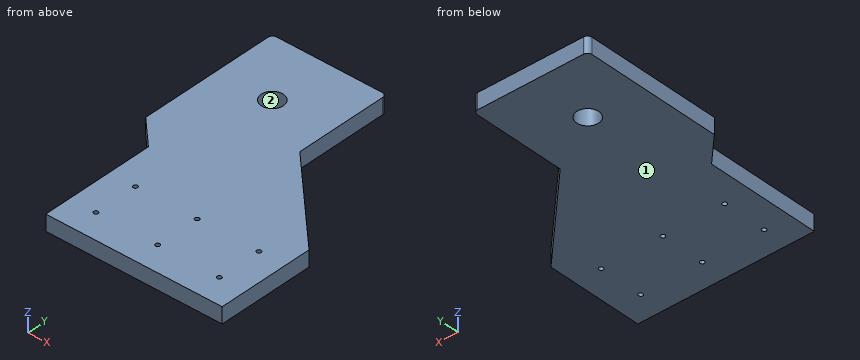
```python
from build123d import *

# Parameters (mm, degrees)
SKETCH1_R                      = 12.5
BOSS_EXTRUDE1_DEPTH            = 18
HOLE_FOR_M5_300_SC_NUTS_SP_1_D = 5


with BuildPart() as part:
    # Sketch1 → Boss-Extrude1 (new body)
    with BuildSketch(Plane.XY):
        with BuildLine():
            Line((4.070181983, 148.487708827), (4.070181983, 43.487708827))
            Line((4.070181983, 43.487708827), (104.070181983, -56.512291173))
            Line((104.070181983, -56.512291173), (104.070181983, -166.512291173))
            Line((104.070181983, -166.512291173), (-95.929818017, -166.512291173))
            Line((-95.929818017, -166.512291173), (-95.929818017, -36.512291173))
            Line((-95.929818017, -36.512291173), (-125.929818017, -6.512291173))
            Line((-125.929818017, -6.512291173), (-125.929818017, 148.487708827))
            ThreePointArc((-125.929818017, 148.487708827), (-124.465351923, 152.023242733), (-120.929818017, 153.487708827))
            Line((-120.929818017, 153.487708827), (-95.929818017, 153.487708827))
            Line((-95.929818017, 153.487708827), (-0.929818017, 153.487708827))
            ThreePointArc((-0.929818017, 153.487708827), (2.605715889, 152.023242733), (4.070181983, 148.487708827))
        make_face()
        with Locations((-62.929818017, 83.487708827)):
            Circle(SKETCH1_R, mode=Mode.SUBTRACT)
    extrude(amount=BOSS_EXTRUDE1_DEPTH)

    # Hole for M5 300® SC Nuts (SP)1 (through all)
    with Locations(Plane.XY.offset(18)):
        with Locations((74.070181983, -86.512291173), (74.070181983, -136.512291173), (4.070181983, -136.512291173), (-65.929818017, -136.512291173), (-65.929818017, -86.512291173), (4.070181983, -86.512291173)):
            Hole(HOLE_FOR_M5_300_SC_NUTS_SP_1_D / 2)


solid = part.part
```
Input: part model. Units: mm. Frame: model coordinates. Face numbers are marked on the shaded views. Give positions to 0.01 mm unless a question says otherwise; leave off trailing zeros. Order: outer loops, then holes, each group sorted by start corner. A loop starts at its lowest first (then second) coordinate and runs counter-clockwise, first axis right, second up. Notation, with made-up numbers: M -37.75,24.5 L -17.75,24.5 A4 cw -17.75,31.5 Z; hole C 13.25,78.25 d6. An arc over 180 degrees is marked long. Return JSON: item names as keys, results as strings.
1) Section query D-D on x = -100.5. Output: boundary loops of the cut face in (y, z), and give its area (3 significant figures).
Taken from the geometry:
{"outline": "M -31.94,0 L 153.49,0 L 153.49,18 L -31.94,18 Z", "area": "3,340 mm2"}
2) Section query C-C on y = -113. Output: boundary loops of the cut face in (x, z).
Taken from the geometry:
{"outline": "M -95.93,0 L 104.07,0 L 104.07,18 L -95.93,18 Z"}
3) Line query: L1, parallel to X at y = -135, z = 11.5; L2, parallel to Y at x = -64, z = 5; L3, parallel to X at y = -71.5, z = 10. Output: solid intervals per line, ascending. Write a range as [from, to].
Taken from the geometry:
{"L1": "x = [-95.93, -67.92], [-63.94, 2.08], [6.06, 72.08], [76.06, 104.07]", "L2": "y = [-166.51, -138.1], [-134.92, -88.1], [-84.92, 71.03], [95.94, 153.49]", "L3": "x = [-95.93, 104.07]"}
4) Section query B-B on z = 10.5. Output: boundary loops of the cut face in (x, y).
Taken from the geometry:
{"outline": "M -125.93,-6.51 L -95.93,-36.51 L -95.93,-166.51 L 104.07,-166.51 L 104.07,-56.51 L 4.07,43.49 L 4.07,148.49 A5 ccw -0.93,153.49 L -120.93,153.49 A5 ccw -125.93,148.49 Z; hole C -62.93,83.49 d25; hole C -65.93,-136.51 d5; hole C -65.93,-86.51 d5; hole C 4.07,-136.51 d5; hole C 4.07,-86.51 d5; hole C 74.07,-136.51 d5; hole C 74.07,-86.51 d5"}
5) Mould query, pull axis X, two halves, no side actions, for the marked faces 1 and 2. Classes: released by +X, released by -X, zero draft, split by the parting line, or undercut.
Taken from the geometry:
{"face 1": "zero draft", "face 2": "undercut"}
6) Contact query for flat-ended pins moving along their axis: pin 1 (15 mm diameter, centred on x = -62.93, y = 83.49, fed in from -Z); pin 2 (1.5 mm diameter, centred on y = 19.5, z = 10, fed in from +X); pin 3 (10 mm diameter, centred on y = -130, z = 9, fed in from -X). Output: stop coordinate, or through.
Taken from the geometry:
{"pin 1": "passes through", "pin 2": "stops at x = 28.81", "pin 3": "stops at x = -95.93"}
7) Section query A-A on y = 87. Output: boundary loops of the cut face in (x, z).
Taken from the geometry:
{"outline": "M -125.93,0 L -74.93,0 L -74.93,18 L -125.93,18 Z; M -50.93,0 L 4.07,0 L 4.07,18 L -50.93,18 Z"}
